```python
from build123d import *

# Parameters (mm, degrees)
SKETCH1_R           = 2.5
SKETCH1_R_2         = 4
BOSS_EXTRUDE1_DEPTH = 5
FILLET1_R           = 10
FILLET2_R           = 10


with BuildPart() as part:
    # Sketch1 → Boss-Extrude1 (new body)
    with BuildSketch(Plane.XY):
        with BuildLine():
            Line((45, 12.742977306), (45, 2.742977306))
            Line((45, 2.742977306), (2.807261435, -9.597879101))
            ThreePointArc((2.807261435, -9.597879101), (0, -10), (-2.807261435, -9.597879101))
            Line((-2.807261435, -9.597879101), (-45, 2.742977306))
            Line((-45, 2.742977306), (-45, 12.742977306))
            ThreePointArc((-45, 12.742977306), (0, 21.5), (45, 12.742977306))
        make_face()
        Circle(SKETCH1_R, mode=Mode.SUBTRACT)
        with Locations((16, 10)):
            Circle(SKETCH1_R_2, mode=Mode.SUBTRACT)
        with Locations((-16, 10)):
            Circle(SKETCH1_R_2, mode=Mode.SUBTRACT)
    extrude(amount=BOSS_EXTRUDE1_DEPTH)

    # Fillet1
    fillet1_edges = [part.edges().sort_by_distance(p)[0] for p in [
        (-45, 2.742977306, 2.5),
        (45, 2.742977306, 2.5),
    ]]
    fillet(fillet1_edges, radius=FILLET1_R)

    # Fillet2
    # the kernel refuses this fillet: 10 mm, written as the material it takes off along each edge
    with BuildSketch(Plane(origin=(45, 12.742977306, -14.490141462), x_dir=(0, -1, 0), z_dir=(0, 0, 1))) as fillet2_piece_1:
        with BuildLine():
            CenterArc((7.397382661, -8.722011181), FILLET2_R, 119.284560105, 41.458809305)
            Line((-2.043125943, -5.424012197), (-2.231936115, -5.358052218))
            ThreePointArc((-2.231936115, -5.358052218), (-1.241477696, -2.629168254), (-0.185404962, 0.075))
            Line((-0.185404962, 0.075), (0, 0.2))
            ThreePointArc((0, 0.2), (1.252954174, 0.2), (2.408078861, 0.174440224))
            Line((2.408078861, 0.174440224), (2.505908347, 0))
        make_face()
    extrude(amount=33.980282925, mode=Mode.SUBTRACT)
    with BuildSketch(Plane(origin=(-45, 12.742977306, -14.490141462), x_dir=(0.9358107737298137, 0.3525027599483545, 0), z_dir=(0, 0, 1))) as fillet2_piece_2:
        with BuildLine():
            CenterArc((5.554554227, -9.997083405), FILLET2_R, 88.616158877, 41.458809305)
            Line((-0.883339609, -2.34505603), (-1.012097485, -2.192015482))
            ThreePointArc((-1.012097485, -2.192015482), (-0.628831959, -1.102027463), (-0.187162155, 0.070500552))
            Line((-0.187162155, 0.070500552), (-0.004830047, 0.199941668))
            ThreePointArc((-0.004830047, 0.199941668), (2.898028292, 0.234999137), (5.800886632, 0.199941668))
            Line((5.800886632, 0.199941668), (5.796056585, 0))
        make_face()
    extrude(amount=33.980282925, mode=Mode.SUBTRACT)


solid = part.part
```
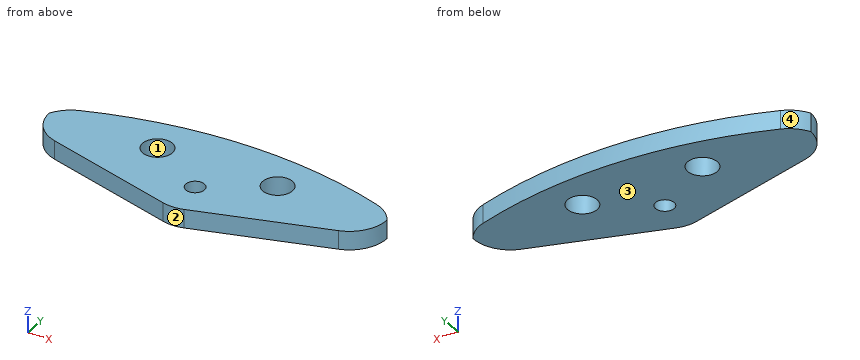
Here's how the part is built. I have some questions about the finished solid (model axes, mm). Face numbers are marked on the shaded views. Round coordinates to 2 decimals unless told otherwise and drop trailing zeros. Loops run counter-clockwise (first coordinate to the right, second up) from the corner with the lowest first, then second, coordinate; pieces in that order, holes last. Notation, with made-up numbers: (-18.5, 13.25) -> (10.5, 13.25) arc R16 cw to (10.5, 28.25) -> close; hole circle Ø11 at (14, 30). An arc over 180 degrees is marked (long way). Answer as CSV lines item,"result". Start each with the question number.
1. Imagine slicing it at D-D on y = 1.5. Write out the boundary of the cut face in (x, z).
2. Imagine slicing it at B-B on x = 0. Write out the boundary of the cut face in (y, z), plus the area to 4 significant figures.
3. Imagine slicing it at C-C on y = 7. Write out the boundary of the cut face in (x, z), plus the area to 3 significant figures.
4. I'm going to push a flat-ended pin straight in: P1, Ø1, axis at x = -14.5, z = 0.5, coming from the +Y side. Where does the tip first touch, or does it pass through?
5. I need wall thicknesses on probe 1 along Y at (x, z) = (0, 3.3); probe 2 along X at (y, z) = (13, 3.2); probe 3 along Y at (x, z) = (16, 1.4). Which ranges of each line are inside material? Lowest first, please. Write a range as from..to.
6. If we mould it in two halves opening along Y, with no side actions, what happens to the marked faces 1, 2, 3 and 4? For each: pulls with the +Y half, pulls with the -Y half, needs draft (parallel to the pull), parting line crosses it, or undercut.
7. Imagine slicing it at A-A on z = 1.6. Write out the boundary of the cut face in (x, y), plus the area to 3 significant figures.
Solution:
1,outline,"(-39.86, 0) -> (-2, 0) -> (-2, 5) -> (-39.86, 5) -> close; (2, 0) -> (39.86, 0) -> (39.86, 5) -> (2, 5) -> close"
2,outline,"(-10, 0) -> (-2.5, 0) -> (-2.5, 5) -> (-10, 5) -> close; (2.5, 0) -> (21.5, 0) -> (21.5, 5) -> (2.5, 5) -> close"
2,area,"132.5 mm²"
3,outline,"(-44.46, 0) -> (-18.65, 0) -> (-18.65, 5) -> (-44.46, 5) -> close; (-13.35, 0) -> (13.35, 0) -> (13.35, 5) -> (-13.35, 5) -> close; (18.65, 0) -> (44.46, 0) -> (44.46, 5) -> (18.65, 5) -> close"
3,area,"392 mm²"
4,P1,"y = 20.68"
5,probe 1,"-10..-2.5, 2.5..21.5"
5,probe 2,"-42.71..-18.65, -13.35..13.35, 18.65..42.71"
5,probe 3,"-5.74..6, 14..20.43"
6,face 1,"undercut"
6,face 2,"pulls with the -Y half"
6,face 3,"needs draft"
6,face 4,"pulls with the +Y half"
7,outline,"(-45, 10.24) arc R10 ccw to (-37.81, 0.64) -> (-2.81, -9.6) arc R10 ccw to (2.81, -9.6) -> (37.81, 0.64) arc R10 ccw to (45, 10.24) arc R10 ccw to (39.58, 14.79) arc R120 ccw to (-39.58, 14.79) arc R10 ccw to start; hole circle Ø8 at (-16, 10); hole circle Ø5 at (0, 0); hole circle Ø8 at (16, 10)"
7,area,"1,870 mm²"
